Answer from the drawing. Dimensions are ordinates in mm from the lowest x, y and z of the part. A direction names the side the tool comes from. Give positions to 0.01 mm unless a question says otherwise; leave off trailing zeros. Loops run counter-clockwise (first coordinate to the right, second up) from the corner with the lowest first, then second, coordinate; pieces in that order, holes last. Notation, with made-up numbers: (6.5, -6.5) - (37.5, -6.5) arc R16 cw to (37.5, 15.5) - close; hole circle Ø8 at (-18.5, 44.5). An arc over 180 degrees is marked (long way). One line per item, written item: value.
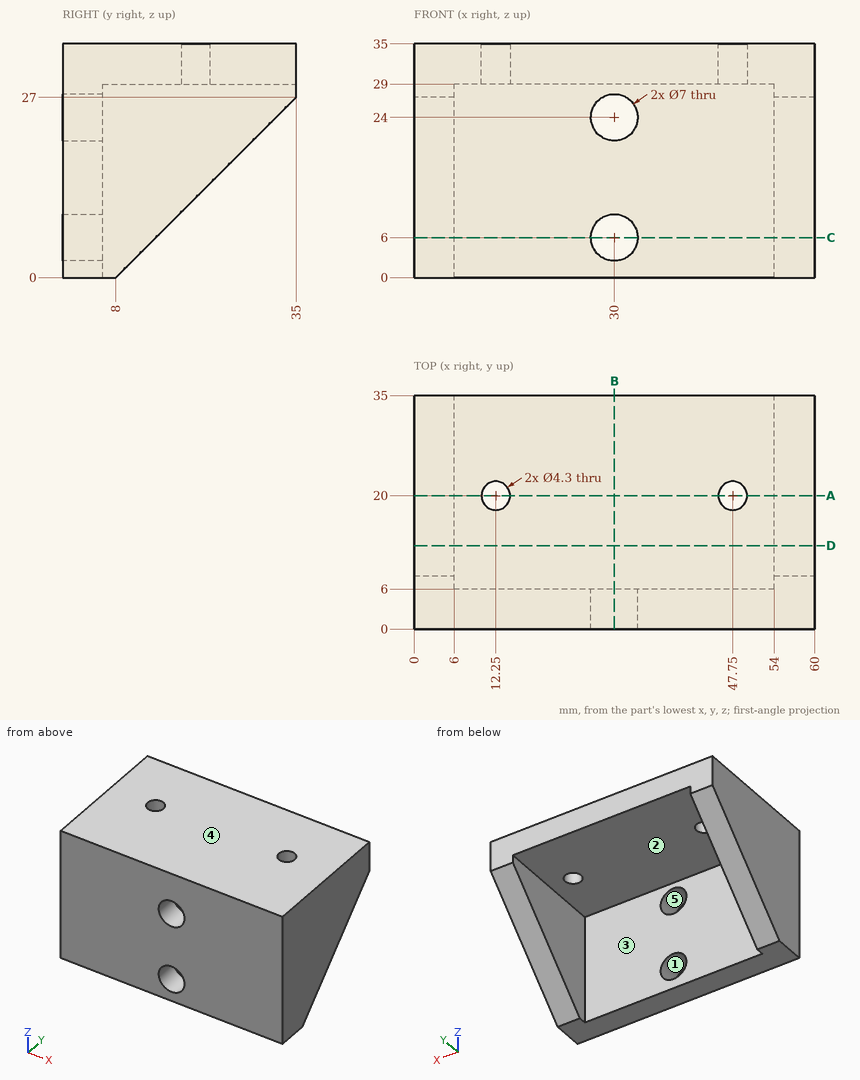
1. Flat-ended cylindrical pins translate along their axes: pin 1 Ø5 at (x, z) = (16.5, 17.5) entering from +Y; pin 2 Ø8.5 at (x, y) = (34, 24) entering from -Z. Find the tip coordinate at first contact, or state that the pin passes through.
Output:
pin 1: stops at y = 6
pin 2: stops at z = 29
2. Section A-A (y = 20) is taken. Write down the section's boundary in (x, z), and give its area (3 significant figures).
Output:
outline: (0, 12) - (6, 12) - (6, 29) - (10.1, 29) - (10.1, 35) - (0, 35) - close; (14.4, 29) - (45.6, 29) - (45.6, 35) - (14.4, 35) - close; (49.9, 29) - (54, 29) - (54, 12) - (60, 12) - (60, 35) - (49.9, 35) - close
area: 512 mm²
3. Find the intervals of material crossed by line 1 along X through (y, z) = (12, 27); line 2 along X through (y, z) = (3, 6); line 3 along Y through (x, z) = (47.75, 31.4), in increasing order.
Output:
line 1: x = 0 to 6, 54 to 60
line 2: x = 0 to 26.5, 33.5 to 60
line 3: y = 0 to 17.85, 22.15 to 35
4. Section B-B (x = 30) is taken. Write down the section's boundary in (y, z), and give its area (3 significant figures).
Output:
outline: (0, 0) - (6, 0) - (6, 2.5) - (0, 2.5) - close; (0, 9.5) - (6, 9.5) - (6, 20.5) - (0, 20.5) - close; (0, 27.5) - (6, 27.5) - (6, 29) - (35, 29) - (35, 35) - (0, 35) - close
area: 300 mm²
5. For the marked faces 1 and 2, determine the directions among +Z, -Z, +X, -X, +Y, -Y from which every point of the face is accessible in a straight line to the end or side of a thin tool.
Output:
face 1: +Y, -Y
face 2: -Z, +Y
6. Section C-C (z = 6) is taken. Write down the section's boundary in (x, y), and give its area (3 significant figures).
Output:
outline: (0, 0) - (26.5, 0) - (26.5, 6) - (6, 6) - (6, 14) - (0, 14) - close; (33.5, 0) - (60, 0) - (60, 14) - (54, 14) - (54, 6) - (33.5, 6) - close
area: 414 mm²
7. Section D-D (y = 12.5) is taken. Write down the section's boundary in (x, z), and give its area (3 significant figures).
Output:
outline: (0, 4.5) - (6, 4.5) - (6, 29) - (54, 29) - (54, 4.5) - (60, 4.5) - (60, 35) - (0, 35) - close
area: 654 mm²
8. The mould has two halves that part along Z. Classify the marked faces 3, 4 and 5: released by +Z, released by -Z, zero draft, split by the parting line, or undercut.
Output:
face 3: zero draft
face 4: released by +Z
face 5: undercut
